Geometry check sheet. Reference: drawing and pictorial views, mm from the part's lowest x, y, z. A direction names the side the tool comes from. Round coordinates to 2 decimals unless told otherwise and drop trailing zeros. Loops run counter-clockwise (first coordinate to the right, second up) from the corner with the lowest first, then second, coordinate; pieces in that order, holes last. Notation, with made-up numbers: (-5, 48.5) -> (32, 48.5) arc R11 ccw to (32, 58.5) -> close; hole circle Ø9 at (59, -3.5). An arc over 180 degrees is marked (long way). Write item = value, one per line.
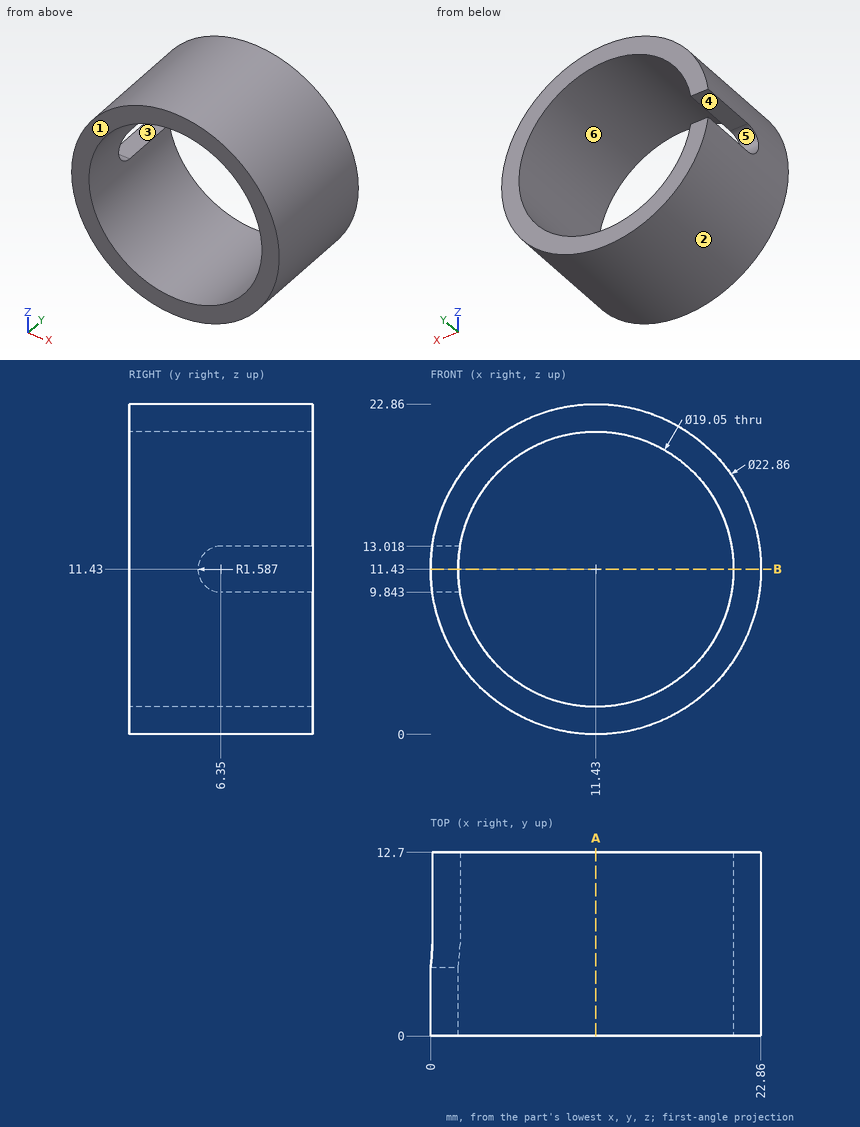
(1) Sectioned sample at A-A, the plane x = 11.43. Record the cut outline in (y, z) (1 decimal).
Filled sheet:
outline = (0, 0) -> (12.7, 0) -> (12.7, 1.9) -> (0, 1.9) -> close; (0, 21) -> (12.7, 21) -> (12.7, 22.9) -> (0, 22.9) -> close
(2) Set-up check for the marked faces 5 and 6: record each of +Z, -Z, +X, -X, +Y, -Y from which the full face is reachable in a straight line by a thin tool's end or side.
Filled sheet:
face_5 = -X, +Y
face_6 = +Y, -Y
(3) Sectioned sample at B-B, the plane z = 11.43. Record the cut outline in (x, y) (1 decimal).
Filled sheet:
outline = (0, 0) -> (1.9, 0) -> (1.9, 4.8) -> (0, 4.8) -> close; (21, 0) -> (22.9, 0) -> (22.9, 12.7) -> (21, 12.7) -> close
(4) Go/stop test with flat-tipped pins: pin 1 Ø1.5 at (x, y) = (1.5, 8) entering from +Z; pin 2 Ø5 at (x, z) = (7, 15.5) entering from +Y; pin 3 Ø0.6 at (x, y) = (1, 11) entering from -Z (1 decimal); pin 4 Ø2 at (x, y) = (15.5, 8) entering from +Z. Record where each tip stops, or that it passes through.
Filled sheet:
pin_1 = 18.24
pin_2 = through
pin_3 = 6.1
pin_4 = 22.44
(5) Material ranges on probe 1 along Z at (x, y) = (11.43, 7) (1 decimal); probe 2 along X at (y, z) = (9.25, 11.43) (1 decimal); probe 3 along X at (y, z) = (11, 13.75), recorded low to high. Write a range as from..to.
Filled sheet:
probe_1 = 0..1.9, 21..22.9
probe_2 = 21..22.9
probe_3 = 0.24..2.19, 20.67..22.62
(6) Draft check along Z on the marked faces 1, 2, 3 and 4. Enter one of: released by +Z, released by -Z, zero draft, split by the parting line, or undercut.
Filled sheet:
face_1 = zero draft
face_2 = split by the parting line
face_3 = undercut
face_4 = undercut
